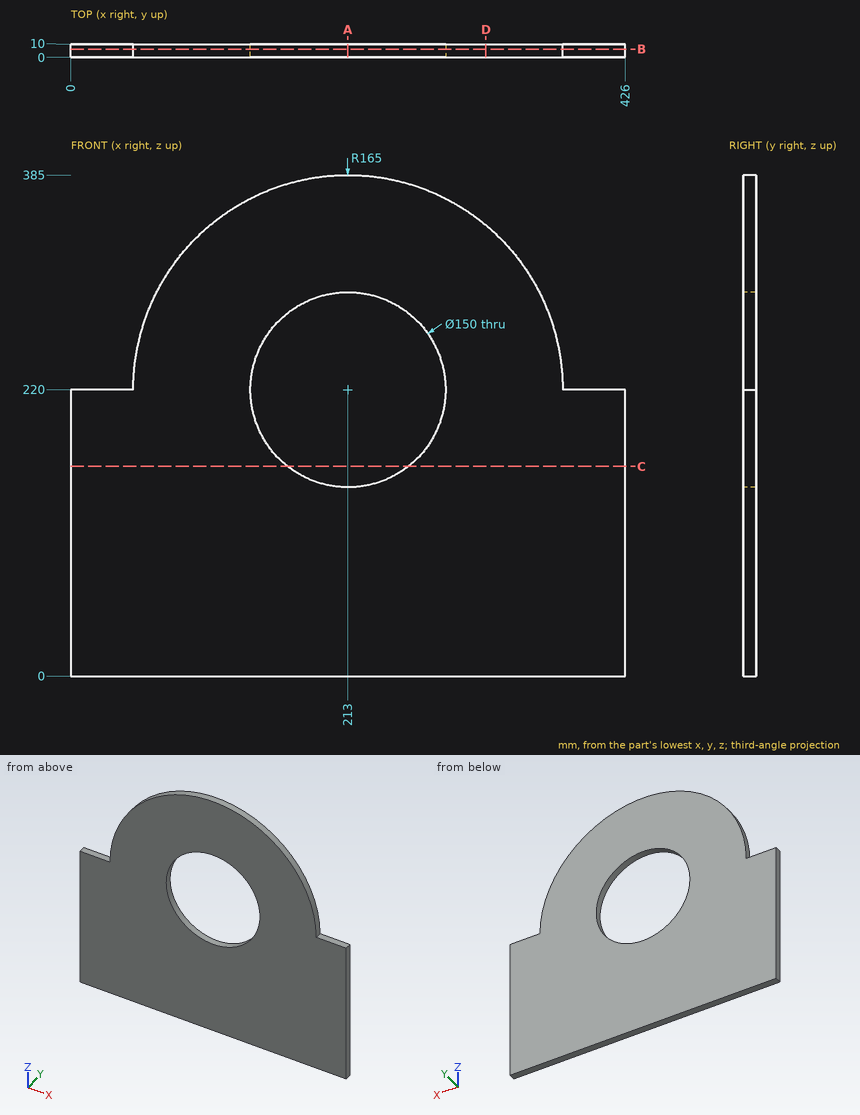
Design review of the part shown in the three views and the two pictorial views. Dimensions are in mm from the part's minimum x, y and z. Coordinates: 2 decimals unless noted, no trailing zeros. Order: outer loops, then holes, each group sorted by start corner. A loop starts at its lowest first (then second) coordinate and runs counter-clockwise, first axis right, second up.
Item 1: For line 1 (Z direction, x = 213, y = 4); line 2 (Z direction, x = 188.5, y = 2.25); line 3 (Z direction, x = 33.5, y = 3.75), list the stretches that pass through material, from the lowest coordinate up.
Item 2: For pin 1 Ø3 at (x, y) = (399.5, 7) entering from +Z; pin 2 Ø6 at (x, y) = (208.5, 8) entering from +Z; pin 3 Ø4 at (x, y) = (251.5, 4) entering from +Z, all flat-tipped, find the tip position at first contact; note any pin that passes through.
Item 3: Take a section at B-B, the plane y = 6. Write out the cut boundary in (x, z).
Item 4: Take a section at C-C, the plane z = 161. Write out the cut boundary in (x, y).
Item 5: Take a section at D-D, the plane x = 319. Write out the cut boundary in (y, z), then the cut area to 3 significant figures.
Item 6: Take a section at A-A, the plane x = 213. Write out the cut boundary in (y, z), then the cut area to 3 significant figures.
The answers:
1. line 1: z = 0 to 145, 295 to 385
1. line 2: z = 0 to 149.11, 290.89 to 383.17
1. line 3: z = 0 to 220
2. pin 1: stops at z = 220
2. pin 2: stops at z = 384.99
2. pin 3: stops at z = 380.91
3. outline: (0, 0) - (426, 0) - (426, 220) - (378, 220) arc R165 ccw to (48, 220) - (0, 220) - close; hole circle Ø150 at (213, 220)
4. outline: (0, 0) - (166.7, 0) - (166.7, 10) - (0, 10) - close; (259.3, 0) - (426, 0) - (426, 10) - (259.3, 10) - close
5. outline: (0, 0) - (10, 0) - (10, 346.45) - (0, 346.45) - close
5. area: 3,460 mm2
6. outline: (0, 0) - (10, 0) - (10, 145) - (0, 145) - close; (0, 295) - (10, 295) - (10, 385) - (0, 385) - close
6. area: 2,350 mm2
